Geometry: see drawing. Coordinates: mm, zero at the bounding-box minimum. A direction names the side the tool comes from. Coordinates: 2 decimals unless noted, no trailing zeros. Loops run counter-clockwise (first coordinate to the right, second up) from the corner with the lowest first, then second, coordinate; pieces in that order, holes last. Notation, with made-up numbers: (-36.75, -20.75) - (-7.75, -20.75) arc R13 cw to (-7.75, -0.75) - close; hole circle Ø8 at (-31.5, 80). An arc over 180 degrees is marked (long way). Answer in a Markdown table with one row per item.
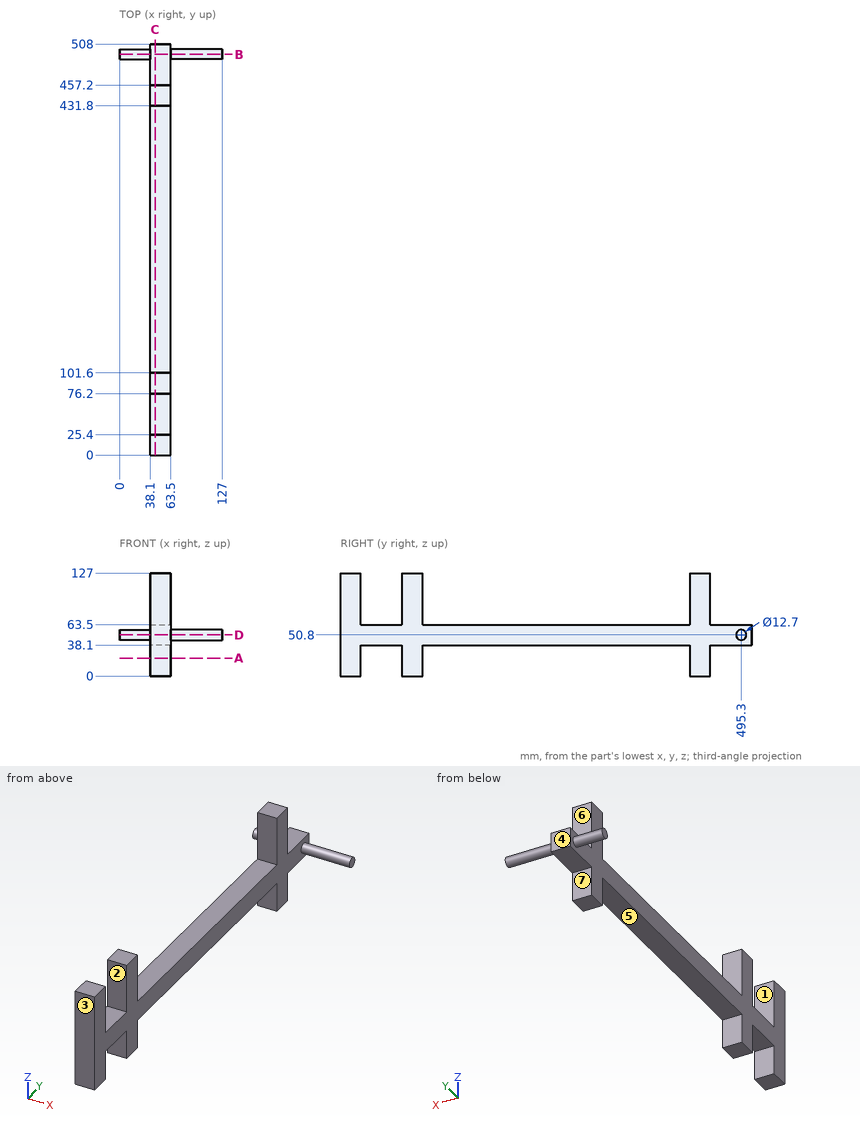
(1) Access query for the marked faces 5, 6 and 7. Directions: +Z, -Z, +X, -X, +Y, -Y. A direction counts if a zero-diameter tool reaches every point of the face in a straight line with its end or side. Return the directions, or none.
Verdict:
| item | result |
|---|---|
| face 5 | -Z, +X, -X |
| face 6 | +Z, +X, -X, +Y |
| face 7 | -Z, +X, -X, +Y |
(2) Cut plane A-A on z = 22. Output: boundary loops of the cut face in (x, y).
Verdict:
| item | result |
|---|---|
| outline | (38.1, 0) - (63.5, 0) - (63.5, 25.4) - (38.1, 25.4) - close; (38.1, 76.2) - (63.5, 76.2) - (63.5, 101.6) - (38.1, 101.6) - close; (38.1, 431.8) - (63.5, 431.8) - (63.5, 457.2) - (38.1, 457.2) - close |
(3) Ray query, probe 1 along Y at (x, z) = (49, 28.5); probe 2 along X at (y, z) = (22.5, 85). Return the intervals inside material, ascending.
Verdict:
| item | result |
|---|---|
| probe 1 | y = 0 to 25.4, 76.2 to 101.6, 431.8 to 457.2 |
| probe 2 | x = 38.1 to 63.5 |
(4) Cut plane C-C on x = 44. Output: boundary loops of the cut face in (y, z), then the cut area to 3 significant figures.
Verdict:
| item | result |
|---|---|
| outline | (0, 0) - (25.4, 0) - (25.4, 38.1) - (76.2, 38.1) - (76.2, 0) - (101.6, 0) - (101.6, 38.1) - (431.8, 38.1) - (431.8, 0) - (457.2, 0) - (457.2, 38.1) - (508, 38.1) - (508, 63.5) - (457.2, 63.5) - (457.2, 127) - (431.8, 127) - (431.8, 63.5) - (101.6, 63.5) - (101.6, 127) - (76.2, 127) - (76.2, 63.5) - (25.4, 63.5) - (25.4, 127) - (0, 127) - close |
| area | 20,600 mm² |
(5) Cut plane B-B on y = 495.3. Output: boundary loops of the cut face in (x, z), then the cut area to 3 significant figures.
Verdict:
| item | result |
|---|---|
| outline | (0, 44.45) - (38.1, 44.45) - (38.1, 38.1) - (63.5, 38.1) - (63.5, 44.45) - (127, 44.45) - (127, 57.15) - (63.5, 57.15) - (63.5, 63.5) - (38.1, 63.5) - (38.1, 57.15) - (0, 57.15) - close |
| area | 1,940 mm² |
(6) Cut plane D-D on z = 50.8. Output: boundary loops of the cut face in (x, y).
Verdict:
| item | result |
|---|---|
| outline | (0, 488.95) - (38.1, 488.95) - (38.1, 0) - (63.5, 0) - (63.5, 488.95) - (127, 488.95) - (127, 501.65) - (63.5, 501.65) - (63.5, 508) - (38.1, 508) - (38.1, 501.65) - (0, 501.65) - close |
(7) Pull-direction query (Y, two-part tool) for the marked faces 1, 2, 3 and 4; classes: pulls with the +Y half, pulls with the -Y half, needs draft (parallel to the pull), parting line crosses it, or undercut.
Verdict:
| item | result |
|---|---|
| face 1 | undercut |
| face 2 | undercut |
| face 3 | pulls with the -Y half |
| face 4 | pulls with the +Y half |
(8) First-contact query: pin 1 Ø5 at (x, y) = (50, 204) entering from -Z; pin 2 Ø6 at (x, z) = (34.5, 42) entering from +Y; pin 3 Ø7.5 at (x, z) = (51, 13) entering from +Y. Flat tips, straight axial feed; report the tip coordinate or a pass-through.
Verdict:
| item | result |
|---|---|
| pin 1 | stops at z = 38.1 |
| pin 2 | stops at y = 497.89 |
| pin 3 | stops at y = 457.2 |
